CAD build for the part. Positions are in the model's coordinates, mm. Coordinates: 2 decimals unless noted, no trailing zeros. Loops run counter-clockwise (first coordinate to the right, second up) from the corner with the lowest first, then second, coordinate; pieces in that order, holes last. Notation, with made-up numbers: M 84,1 L 100,1 A32 ccw 100,32 Z; hole C 37,57.25 d8. An arc over 180 degrees is marked long. Answer as a JSON object with one key per item and string values. Group by question number.
```python
from build123d import *

# Parameters (mm, degrees)
F0_R     = 1.6
F1_DEPTH = 3.175


# Not quite as in the source:
# - a length typed as a fraction of an inch, garbled in the dataset ("3 / 203.2 mm" for 3/8 in), is restored


with BuildPart() as f1:
    # F0 (on Front) → F1 (new body)
    with BuildSketch(Plane.XZ):
        with BuildLine():
            Line((57.46, 0), (2.54, 0))
            ThreePointArc((2.54, 0), (0.7439487758, -0.7439487758), (0, -2.54))
            Line((0, -2.54), (0, -27.46))
            ThreePointArc((0, -27.46), (0.7439487758, -29.2560512242), (2.54, -30))
            Line((2.54, -30), (57.46, -30))
            ThreePointArc((57.46, -30), (59.2560512242, -29.2560512242), (60, -27.46))
            Line((60, -27.46), (60, -2.54))
            ThreePointArc((60, -2.54), (59.2560512242, -0.7439487758), (57.46, 0))
        make_face()
        with Locations((5, -25)):
            Circle(F0_R, mode=Mode.SUBTRACT)
        with Locations((15, -25)):
            Circle(F0_R, mode=Mode.SUBTRACT)
        with Locations((25, -25)):
            Circle(F0_R, mode=Mode.SUBTRACT)
        with Locations((35, -25)):
            Circle(F0_R, mode=Mode.SUBTRACT)
        with Locations((45, -25)):
            Circle(F0_R, mode=Mode.SUBTRACT)
        with Locations((55, -25)):
            Circle(F0_R, mode=Mode.SUBTRACT)
        with Locations((5, -15)):
            Circle(F0_R, mode=Mode.SUBTRACT)
        with Locations((15, -15)):
            Circle(F0_R, mode=Mode.SUBTRACT)
        with Locations((25, -15)):
            Circle(F0_R, mode=Mode.SUBTRACT)
        with Locations((5, -5)):
            Circle(F0_R, mode=Mode.SUBTRACT)
        with Locations((15, -5)):
            Circle(F0_R, mode=Mode.SUBTRACT)
        with Locations((25, -5)):
            Circle(F0_R, mode=Mode.SUBTRACT)
        with Locations((35, -15)):
            Circle(F0_R, mode=Mode.SUBTRACT)
        with Locations((45, -15)):
            Circle(F0_R, mode=Mode.SUBTRACT)
        with Locations((55, -15)):
            Circle(F0_R, mode=Mode.SUBTRACT)
        with Locations((35, -5)):
            Circle(F0_R, mode=Mode.SUBTRACT)
        with Locations((45, -5)):
            Circle(F0_R, mode=Mode.SUBTRACT)
        with Locations((55, -5)):
            Circle(F0_R, mode=Mode.SUBTRACT)
    extrude(amount=F1_DEPTH)


solid = f1.part
```
Item 1: Slice it at B-B, the plane y = -2.1. Count the separate pieces of the cut face and the enclosed holes in it, then the cut area to 3 significant figures.
Item 2: Drill centre lines: L1, parallel to Z at x = 5, y = -2.35; L2, parallel to Z at x = 14, y = -0.35; L3, parallel to X at y = -0.75, z = -2. Where is each one in solid material? Low to high. Write a range as from..to.
Item 3: Slice it at C-C, the plane z = -15. Write the cut outline in (x, y) (3 decimals).
Item 4: Pin check, flat tip, straight feed: pin 1 (4 mm diameter, centred on x = 13.5, z = -14.5, fed in from +Y). Stop position of the tip, or through.
Item 5: Slice it at A-A, the plane x = 25. Write the cut outline in (y, z) (3 decimals), then the cut area to 3 significant figures.
Item 6: Pull direction X, two halves, no side cores. Call faces 1 (the cylindrical face through (0.764, -1.565, -0.724)), 2 (the cylindrical face through (56.526, -1.565, -24.519)), 3 (the flat face through (60, -2, -15)): released by +X, released by -X, zero draft, split by the parting line, or undercut.
Computed:
{
 "1": {"separate pieces": "1", "enclosed holes": "18", "area": "1,650 mm2"},
 "2": {"L1": "-30..-26.6, -23.4..-16.6, -13.4..-6.6, -3.4..0", "L2": "-30..-26.25, -23.75..-16.25, -13.75..-6.25, -3.75..0", "L3": "0.06..59.94"},
 "3": {"outline": "M 0,-3.175 L 3.4,-3.175 L 3.4,0 L 0,0 Z; M 6.6,-3.175 L 13.4,-3.175 L 13.4,0 L 6.6,0 Z; M 16.6,-3.175 L 23.4,-3.175 L 23.4,0 L 16.6,0 Z; M 26.6,-3.175 L 33.4,-3.175 L 33.4,0 L 26.6,0 Z; M 36.6,-3.175 L 43.4,-3.175 L 43.4,0 L 36.6,0 Z; M 46.6,-3.175 L 53.4,-3.175 L 53.4,0 L 46.6,0 Z; M 56.6,-3.175 L 60,-3.175 L 60,0 L 56.6,0 Z"},
 "4": {"pin 1": "y = 0"},
 "5": {"outline": "M -3.175,-30 L 0,-30 L 0,-26.6 L -3.175,-26.6 Z; M -3.175,-23.4 L 0,-23.4 L 0,-16.6 L -3.175,-16.6 Z; M -3.175,-13.4 L 0,-13.4 L 0,-6.6 L -3.175,-6.6 Z; M -3.175,-3.4 L 0,-3.4 L 0,0 L -3.175,0 Z", "area": "64.8 mm2"},
 "6": {"face 1": "released by -X", "face 2": "undercut", "face 3": "released by +X"}
}
